from build123d import *

# Parameters (mm, degrees)
ESQUISSE1_R             = 30
BOSS_EXTRU_1_DEPTH      = 2
ENL_V_MAT_EXTRU_1_REACH = 185.586
ESQUISSE2_R             = 2.25
ESQUISSE2_R_2           = 2.1
ESQUISSE4_R             = 2
GOUJON_M4X20_DEPTH      = 20


with BuildPart() as part:
    # Esquisse1 → Boss.-Extru.1 (new body)
    with BuildSketch(Plane.XY):
        with BuildLine():
            Line((-90, -160), (90, -160))
            Line((90, -160), (90, 0))
            ThreePointArc((90, 0), (0, 90), (-90, 0))
            Line((-90, 0), (-90, -160))
        make_face()
        Circle(ESQUISSE1_R, mode=Mode.SUBTRACT)
    extrude(amount=BOSS_EXTRU_1_DEPTH)

    # Esquisse2 → Enl_v. mat.-Extru.1 (cut, up to next)
    with BuildSketch(Plane.XY.offset(2), mode=Mode.PRIVATE) as enl_v_mat_extru_1_sk1:
        with Locations((26.162950904, 26.162950904)):
            Circle(ESQUISSE2_R)
    enl_v_mat_extru_1_tool1 = extrude(enl_v_mat_extru_1_sk1.sketch, amount=-ENL_V_MAT_EXTRU_1_REACH, mode=Mode.PRIVATE) & part.part
    # Esquisse2 → Enl_v. mat.-Extru.1 (cut, up to next)
    with BuildSketch(Plane.XY.offset(2), mode=Mode.PRIVATE) as enl_v_mat_extru_1_sk2:
        with Locations((-26.162950904, -26.162950904)):
            Circle(ESQUISSE2_R)
    enl_v_mat_extru_1_tool2 = extrude(enl_v_mat_extru_1_sk2.sketch, amount=-ENL_V_MAT_EXTRU_1_REACH, mode=Mode.PRIVATE) & part.part
    # Esquisse2 → Enl_v. mat.-Extru.1 (cut, up to next)
    with BuildSketch(Plane.XY.offset(2), mode=Mode.PRIVATE) as enl_v_mat_extru_1_sk3:
        with Locations((-26.162950904, 26.162950904)):
            Circle(ESQUISSE2_R)
    enl_v_mat_extru_1_tool3 = extrude(enl_v_mat_extru_1_sk3.sketch, amount=-ENL_V_MAT_EXTRU_1_REACH, mode=Mode.PRIVATE) & part.part
    # Esquisse2 → Enl_v. mat.-Extru.1 (cut, up to next)
    with BuildSketch(Plane.XY.offset(2), mode=Mode.PRIVATE) as enl_v_mat_extru_1_sk4:
        with Locations((26.162950904, -26.162950904)):
            Circle(ESQUISSE2_R)
    enl_v_mat_extru_1_tool4 = extrude(enl_v_mat_extru_1_sk4.sketch, amount=-ENL_V_MAT_EXTRU_1_REACH, mode=Mode.PRIVATE) & part.part
    # Esquisse2 → Enl_v. mat.-Extru.1 (cut, up to next)
    with BuildSketch(Plane.XY.offset(2), mode=Mode.PRIVATE) as enl_v_mat_extru_1_sk5:
        with Locations((0, 37)):
            Circle(ESQUISSE2_R_2)
    enl_v_mat_extru_1_tool5 = extrude(enl_v_mat_extru_1_sk5.sketch, amount=-ENL_V_MAT_EXTRU_1_REACH, mode=Mode.PRIVATE) & part.part
    # Esquisse2 → Enl_v. mat.-Extru.1 (cut, up to next)
    with BuildSketch(Plane.XY.offset(2), mode=Mode.PRIVATE) as enl_v_mat_extru_1_sk6:
        with Locations((0, -37)):
            Circle(ESQUISSE2_R_2)
    enl_v_mat_extru_1_tool6 = extrude(enl_v_mat_extru_1_sk6.sketch, amount=-ENL_V_MAT_EXTRU_1_REACH, mode=Mode.PRIVATE) & part.part
    add(enl_v_mat_extru_1_tool1.solids().sort_by_distance((26.162951, 26.162951, 2))[0], mode=Mode.SUBTRACT)
    add(enl_v_mat_extru_1_tool2.solids().sort_by_distance((-26.162951, -26.162951, 2))[0], mode=Mode.SUBTRACT)
    add(enl_v_mat_extru_1_tool3.solids().sort_by_distance((-26.162951, 26.162951, 2))[0], mode=Mode.SUBTRACT)
    add(enl_v_mat_extru_1_tool4.solids().sort_by_distance((26.162951, -26.162951, 2))[0], mode=Mode.SUBTRACT)
    add(enl_v_mat_extru_1_tool5.solids().sort_by_distance((0, 37, 2))[0], mode=Mode.SUBTRACT)
    add(enl_v_mat_extru_1_tool6.solids().sort_by_distance((0, -37, 2))[0], mode=Mode.SUBTRACT)

    # Esquisse4 → Goujon M4x20 (add)
    with BuildSketch(Plane(origin=(0, 0, 0), x_dir=(-1, 0, 0), z_dir=(0, 0, -1))):
        with Locations(Location((-20, -100, 0), (0, 0, 180))):
            Circle(ESQUISSE4_R)
        with Locations(Location((20, -100, 0), (0, 0, 180))):
            Circle(ESQUISSE4_R)
    extrude(amount=GOUJON_M4X20_DEPTH)


solid = part.part
Read the model definition and answer for the solid it produces. Units are mm, in the model's axes. Give positions to 0.01 mm unless a question says otherwise; leave off trailing zeros. Write each loop counter-clockwise with the first axis right and the second up, starting at its lowest first coordinate (ties: lowest second). Pieces come first, ordered by that corner, then holes. Notation, with made-up numbers: (80.5, 49) - (114.5, 49) arc R28 cw to (114.5, 82) - close; hole circle Ø11 at (49.25, 52.25). An arc over 180 degrees is marked (long way). Return JSON: item names as keys, results as strings.
Q1. A cutting plane is placed at B-B, the plane y = -18.5. Determine the outline of the cut face in (x, z), and give its area (3 significant figures).
Reply:
{"outline": "(-90, 0) - (-23.62, 0) - (-23.62, 2) - (-90, 2) - close; (23.62, 0) - (90, 0) - (90, 2) - (23.62, 2) - close", "area": "266 mm²"}
Q2. A cutting plane is placed at A-A, the plane z = -17.25. Determine the outline of the cut face in (x, y), and give its area (3 significant figures).
Reply:
{"outline": "circle Ø4 at (-20, -100); circle Ø4 at (20, -100)", "area": "25.1 mm²"}
Q3. Consider line 1 along Y through (x, z) = (0, 1.55); line 2 along Z through (x, y) = (31, -131.5). Determine where each line is inside the solid, lowest interval first. Write a range as [from, to].
Reply:
{"line 1": "[-160, -39.1], [-34.9, -30], [30, 34.9], [39.1, 90]", "line 2": "[0, 2]"}
Q4. A cutting plane is placed at D-D, the plane x = -66. Determine the outline of the cut face in (y, z).
Reply:
{"outline": "(-160, 0) - (61.19, 0) - (61.19, 2) - (-160, 2) - close"}
Q5. A cutting plane is placed at C-C, the plane y = -56. Determine the outline of the cut face in (x, z).
Reply:
{"outline": "(-90, 0) - (90, 0) - (90, 2) - (-90, 2) - close"}
Q6. Given P1, Ø5, axis at x = -60, y = 4.5, coming from the -Z side; P2, Ø4, axis at x = 0, y = 37, coming from the -Z side; P3, Ø7, axis at x = -26.16, y = 26.16, coming from the +Z side, each flat-ended and moving along its own axis, determine where each tip first touches the part or whether it passes through.
Reply:
{"P1": "z = 0", "P2": "through", "P3": "z = 2"}
